Input: dimensioned drawing with shaded views. Units: mm. Origin: part minimum x, y, z. A direction names the side the tool comes from. Coordinates: 2 decimals unless noted, no trailing zeros. Order: outer loops, then holes, each group sorted by start corner. A loop starts at its lowest first (then second) coordinate and runs counter-clockwise, first axis right, second up. Notation, with made-up numbers: (48, -11.75) - (88, -11.75) arc R13 cw to (88, 11.25) - close; hole circle Ø3 at (37, -19). An arc over 180 degrees is marked (long way). Use one line per item in the form item = value. Start each with the question number.
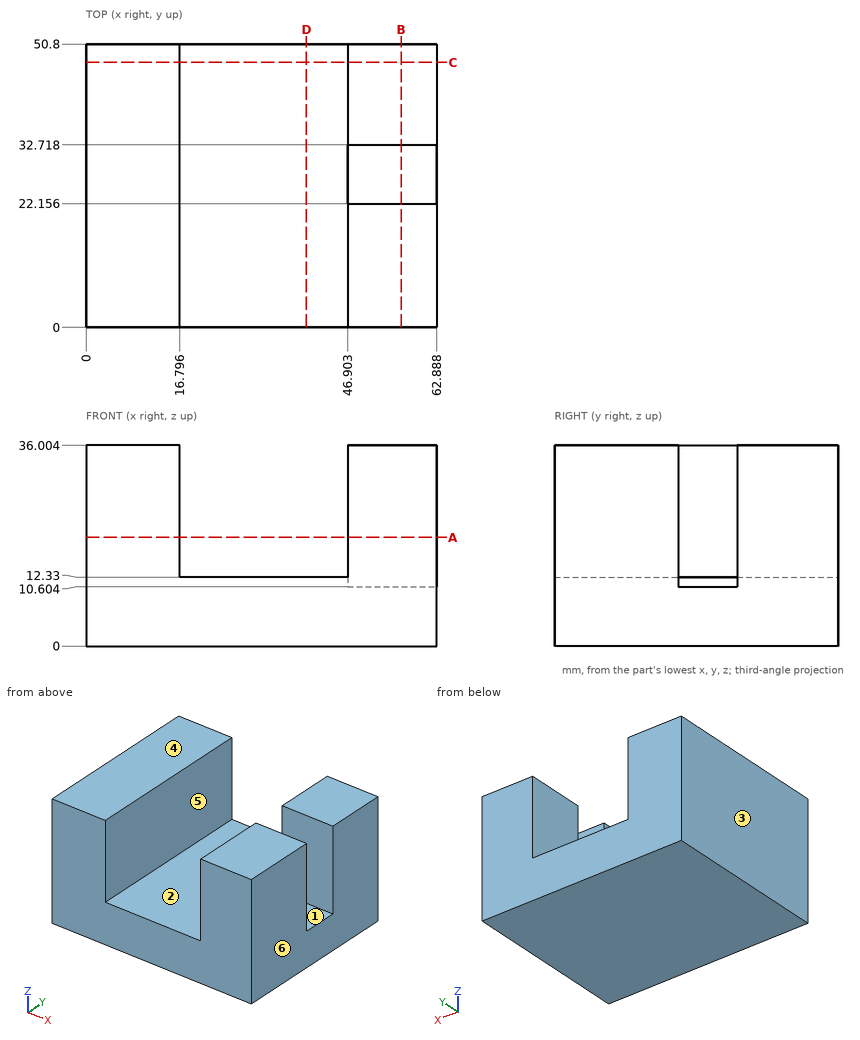
(1) Cut plane D-D on x = 39.5. Return the cut outline in (y, z).
(2) Contact query for flat-ended pins moving along their axis: pin 1 Ø1.4 at (y, z) = (30, 11.5) entering from +X; pin 2 Ø24 at (x, y) = (34.5, 28) entering from +Z. Output: stop coordinate, or through.
(3) Cut plane A-A on z = 19.5. Return the cut outline in (x, y).
(4) Cut plane C-C on y = 47.5. Return the cut outline in (x, z) (1 decimal).
(5) Draft query along X for the marked faces 4, 5 and 6. Return one class per face: released by +X, released by -X, zero draft, split by the parting line, or undercut.
(6) Material intervals for L1, parallel to Y at x = 60, z = 34.5; L2, parallel to X at y = 46, z = 19; L3, parallel to Z at x = 46, y = 5.5, sorted ascending. Write a range as from..to.
(7) Set-up query: the marked faces 1, 2 and 3. Return all of +Z, -Z, +X, -X, +Y, -Y with unobstructed straight access to the full face (end or side cutting, diameter ignored); none if empty.
(8) Cut plane B-B on x = 56.5. Return the cut outline in (y, z) (1 decimal), plus the area to 3 significant figures.
Check sheet entries:
q1.outline = (0, 0) - (50.8, 0) - (50.8, 12.33) - (0, 12.33) - close
q2.pin_1 = 46.9
q2.pin_2 = 12.33
q3.outline = (0, 0) - (16.8, 0) - (16.8, 50.8) - (0, 50.8) - close; (46.9, 0) - (62.89, 0) - (62.89, 22.16) - (46.9, 22.16) - close; (46.9, 32.72) - (62.89, 32.72) - (62.89, 50.8) - (46.9, 50.8) - close
q4.outline = (0, 0) - (62.9, 0) - (62.9, 36) - (46.9, 36) - (46.9, 12.3) - (16.8, 12.3) - (16.8, 36) - (0, 36) - close
q5.face_4 = zero draft
q5.face_5 = undercut
q5.face_6 = released by +X
q6.L1 = 0..22.16, 32.72..50.8
q6.L2 = 0..16.8, 46.9..62.89
q6.L3 = 0..12.33
q7.face_1 = +Z, +X
q7.face_2 = +Z, +Y, -Y
q7.face_3 = +Z, -Z, -X, +Y, -Y
q8.outline = (0, 0) - (50.8, 0) - (50.8, 36) - (32.7, 36) - (32.7, 10.6) - (22.2, 10.6) - (22.2, 36) - (0, 36) - close
q8.area = 1,560 mm^2
